Can you work these out from the model? Positions are in its coordinate system, mm. A direction names the side the tool comes from. Coordinates: 2 decimals unless noted, no trailing zeros. Write each loop counter-clockwise with the first axis right and the second up, starting at its lowest first coordinate (ties: lowest second). Pieces come first, ordered by that corner, then holes. Notation, with made-up numbers: (-32.75, 44.25) -> (0.25, 44.25) arc R18 cw to (0.25, 74.25) -> close; hole circle Ø1 at (41.25, 74). An arc over 180 degrees is marked (long way). Use one line per item in the form item = value.
```python
from build123d import *

# Parameters (mm, degrees)
F4_DEPTH        = 3.175
F4_COPIES_COUNT = 48


# Not quite as in the source:
# - a pattern or mirror of a feature is missing from the dataset's text; its kind, count and spacing are read off the source's solid


with BuildPart() as f2:
    # F1 (on offset) → F2 (revolve)
    with BuildSketch(Plane.XZ.offset(60.325)):
        with BuildLine():
            Line((19.05, 5.762625), (19.05, 1.5875))
            Line((19.05, 1.5875), (27.78125, 1.5875))
            Line((27.78125, 1.5875), (27.78125, 6.35))
            Line((27.78125, 6.35), (24.60625, 6.35))
            Line((24.60625, 6.35), (24.60625, 5.762625))
            ThreePointArc((24.60625, 5.762625), (22.4155, 3.571875), (20.22475, 5.762625))
            Line((20.22475, 5.762625), (19.05, 5.762625))
        make_face()
    revolve(axis=Axis((0, -60.325, 0), (1, 0, 0)))

    # F3 (on face) → F4 (cut, through all)
    with BuildSketch(Plane.YZ.offset(27.78125)):
        with BuildLine():
            ThreePointArc((-59.4961586794, 6.2956748697), (-59.9096901294, 6.3364041626), (-60.325, 6.35))
            Line((-60.325, 6.35), (-59.9371006784, 5.9182))
            Line((-59.9371006784, 5.9182), (-59.4961586794, 6.2956748697))
        make_face()
    f4 = extrude(amount=-F4_DEPTH, mode=Mode.SUBTRACT)

    # F4_copies: F4 ×48 about axis
    f4_copies_axis = Axis((0, -60.325, 0), (1, 0, 0))
    for i in range(1, F4_COPIES_COUNT):
        add(f4.rotate(f4_copies_axis, i * 360 / F4_COPIES_COUNT), mode=Mode.SUBTRACT)


solid = f2.part
```
Q1. Will these pins go through, and if not, where does the flat tip stop? pin 1 (2.5 mm diameter, centred on y = -60.325, z = 0, fed in from +X); pin 2 (4 mm diameter, centred on x = 23.5, y = -57.5, fed in from -Z); pin 3 (4 mm diameter, centred on x = 27, z = 4, fed in from +Y); pin 4 (5 mm diameter, centred on x = 25.5, z = -3, fed in from +Y).
Return value:
pin_1 = through
pin_2 = -6.13
pin_3 = -54.46
pin_4 = -54.03
Q2. If I drill on line 1 (Y direction, x = 21.25, z = 0); line 2 (Y direction, x = 26.25, z = 6); line 3 (Z direction, x = 25.25, y = -66), over which ranges is the centre line in solid material (lowest first)? Write a range as from..to.
Return value:
line_1 = -64.23..-61.91, -58.74..-56.42
line_2 = -62.04..-61.76, -61.36..-60.81, -60.64..-60.01, -59.84..-59.29, -58.89..-58.61
line_3 = -2.5..-2.03, -1.88..1.88, 2.03..2.5
Q3. For faces 1 (the cylindrical face through (19.63, -54.7, -1.25)), 2 (the flat face through (27.781, -59, -1.3)), which set-ups out of +Z, -Z, +X, -X, +Y, -Y let a thin tool reach every point of the face, with its end or its side?
Return value:
face_1 = -X
face_2 = +Z, -Z, +X, +Y, -Y
Q4. Suppose I cut it at A-A (x = 24.25). Write out the boundary of the cut face in (y, z) (1 decimal), then the cut area to 3 significant figures.
Return value:
outline = circle Ø9.1 at (-60.3, 0); hole circle Ø3.2 at (-60.3, 0)
area = 57.6 mm2
Q5. Suppose I cut it at B-B (x = 20.5). Write out the boundary of the cut face in (y, z) (1 decimal), then the cut area to 3 significant figures.
Return value:
outline = circle Ø9.4 at (-60.3, 0); hole circle Ø3.2 at (-60.3, 0)
area = 61.5 mm2
